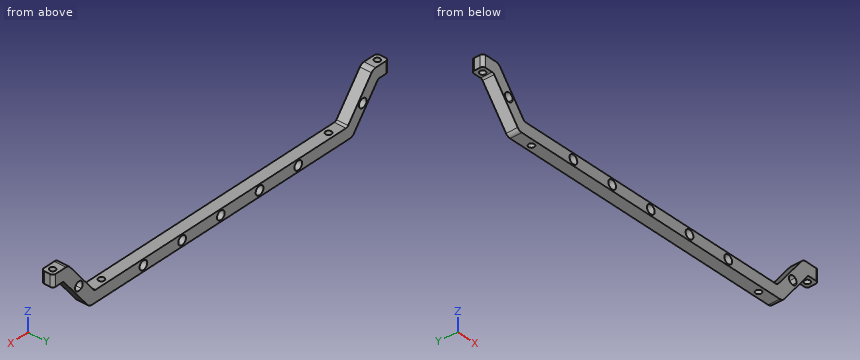
```python
from build123d import *

# Parameters (mm, degrees)
F0_R     = 7.5
F1_DEPTH = 10
F2_R     = 5
F5_D     = 10


with BuildPart() as f1:
    # F0 (on Front) → F1 (new body, symmetric)
    with BuildSketch(Plane.XZ):
        with BuildLine():
            Line((0, 10), (-245.075985, 10))
            Line((-245.075985, 10), (-242.07376, 6.097108))
            ThreePointArc((-242.07376, 6.097108), (-241.028627, -4.417518), (-250, -10))
            Line((-250, -10), (0, -10))
            Line((0, -10), (250, -10))
            ThreePointArc((250, -10), (241.028627, -4.417518), (242.07376, 6.097108))
            Line((242.07376, 6.097108), (245.075985, 10))
            Line((245.075985, 10), (0, 10))
        make_face()
        with Locations((-150, 0)):
            Circle(F0_R, mode=Mode.SUBTRACT)
        with BuildLine():
            ThreePointArc((-82.5, 0), (-75, 7.5), (-67.5, 0))
            ThreePointArc((-67.5, 0), (-75, -7.5), (-82.5, 0))
        make_face(mode=Mode.SUBTRACT)
        with BuildLine():
            ThreePointArc((7.5, 0), (0, -7.5), (-7.5, 0))
            ThreePointArc((-7.5, 0), (0, 7.5), (7.5, 0))
        make_face(mode=Mode.SUBTRACT)
        with BuildLine():
            ThreePointArc((82.5, 0), (75, -7.5), (67.5, 0))
            ThreePointArc((67.5, 0), (75, 7.5), (82.5, 0))
        make_face(mode=Mode.SUBTRACT)
        with BuildLine():
            ThreePointArc((157.5, 0), (150, -7.5), (142.5, 0))
            ThreePointArc((142.5, 0), (150, 7.5), (157.5, 0))
        make_face(mode=Mode.SUBTRACT)
        with BuildLine():
            ThreePointArc((-300, 75), (-308.971373, 69.417518), (-307.92624, 58.902892))
            Line((-307.92624, 58.902892), (-304.924015, 55))
            Line((-304.924015, 55), (-257.92624, -6.097108))
            ThreePointArc((-257.92624, -6.097108), (-254.417518, -8.971373), (-250, -10))
            ThreePointArc((-250, -10), (-241.028627, -4.417518), (-242.07376, 6.097108))
            Line((-242.07376, 6.097108), (-245.075985, 10))
            Line((-245.075985, 10), (-292.07376, 71.097108))
            ThreePointArc((-292.07376, 71.097108), (-295.582482, 73.971373), (-300, 75))
        make_face()
        with BuildLine():
            ThreePointArc((-270.427169, 26.55532), (-280.94468, 27.927169), (-279.572831, 38.44468))
            ThreePointArc((-279.572831, 38.44468), (-271.686862, 39.22853), (-267.5, 32.5))
            ThreePointArc((-267.5, 32.5), (-268.27147, 29.186862), (-270.427169, 26.55532))
        make_face(mode=Mode.SUBTRACT)
        with BuildLine():
            Line((-304.924015, 55), (-307.92624, 58.902892))
            ThreePointArc((-307.92624, 58.902892), (-308.971373, 69.417518), (-300, 75))
            Line((-300, 75), (-320, 75))
            Line((-320, 75), (-325.074017, 75))
            Line((-325.074017, 75), (-325.074017, 55))
            Line((-325.074017, 55), (-320, 55))
            Line((-320, 55), (-319.222152, 55))
            Line((-319.222152, 55), (-304.924015, 55))
        make_face()
        with BuildLine():
            Line((292.07376, 71.097108), (245.075985, 10))
            Line((245.075985, 10), (242.07376, 6.097108))
            ThreePointArc((242.07376, 6.097108), (241.028627, -4.417518), (250, -10))
            ThreePointArc((250, -10), (254.417518, -8.971373), (257.92624, -6.097108))
            Line((257.92624, -6.097108), (304.924015, 55))
            Line((304.924015, 55), (307.92624, 58.902892))
            ThreePointArc((307.92624, 58.902892), (308.971373, 69.417518), (300, 75))
            ThreePointArc((300, 75), (295.582482, 73.971373), (292.07376, 71.097108))
        make_face()
        with BuildLine():
            ThreePointArc((279.572831, 38.44468), (281.72853, 35.813138), (282.5, 32.5))
            ThreePointArc((282.5, 32.5), (278.313138, 25.77147), (270.427169, 26.55532))
            ThreePointArc((270.427169, 26.55532), (269.05532, 37.072831), (279.572831, 38.44468))
        make_face(mode=Mode.SUBTRACT)
        with BuildLine():
            Line((320, 75), (300, 75))
            ThreePointArc((300, 75), (308.971373, 69.417518), (307.92624, 58.902892))
            Line((307.92624, 58.902892), (304.924015, 55))
            Line((304.924015, 55), (319.222152, 55))
            Line((319.222152, 55), (320, 55))
            Line((320, 55), (325.074017, 55))
            Line((325.074017, 55), (325.074017, 75))
            Line((325.074017, 75), (320, 75))
        make_face()
    extrude(amount=F1_DEPTH, both=True)

    # F2
    f2_edges = [f1.edges().sort_by_distance(p)[0] for p in [
        (-245.075985, 0, 10),
        (245.075985, 0, 10),
        (-304.924015, 0, 55),
        (-325.074017, 10, 65),
        (325.074017, -10, 65),
        (325.074017, 10, 65),
        (-325.074017, -10, 65),
    ]]
    fillet(f2_edges, radius=F2_R)

    # F5 (through all)
    with Locations(Plane(origin=(0, 0, -10), x_dir=(1, 0, 0), z_dir=(0, 0, -1))):
        with Locations((-220, 0), (220, 0), (314.522654, 0), (-314.522654, 0)):
            Hole(F5_D / 2)


solid = f1.part
```
Design review of the part built by this model. Coordinates are the model's own, in mm. Coordinates: 2 decimals unless noted, no trailing zeros. Write each loop counter-clockwise with the first axis right and the second up, starting at its lowest first coordinate (ties: lowest second). Pieces come first, ordered by that corner, then holes.
1) Add section A-A (z = 0). Write out the cut boundary in (x, y), plus the area to 3 significant figures.
2) To check wall thickness, follow L1, parallel to Z at x = 75, y = 3.75; L2, parallel to Y at x = 220, z = -1; L3, parallel to X at y = -6.5, z = 2. State the ranges of each line that lie inside material, in increasing order.
3) Insertion check: pin 1 (4 mm diameter, centred on y = -4, z = 17.5, fed in from -X); pin 2 (10 mm diameter, centred on x = 319.5, y = 2, fed in from -Z); pin 3 (8 mm diameter, centred on x = -17.5, y = -7.5, fed in from +Z). Each pin has a flat end and moves straight along its axis. Give the tip position at first contact, or say it passes through.
4) Add section B-B (x = 150). Write out the cut boundary in (y, z), plus the area to 3 significant figures.
Check result:
1. outline: (-262.62, -10) - (-157.5, -10) - (-157.5, 10) - (-262.62, 10) - close; (-142.5, -10) - (-82.5, -10) - (-82.5, 10) - (-142.5, 10) - close; (-67.5, -10) - (-7.5, -10) - (-7.5, 10) - (-67.5, 10) - close; (7.5, -10) - (67.5, -10) - (67.5, 10) - (7.5, 10) - close; (82.5, -10) - (142.5, -10) - (142.5, 10) - (82.5, 10) - close; (157.5, -10) - (262.62, -10) - (262.62, 10) - (157.5, 10) - close; hole circle Ø10 at (-220, 0); hole circle Ø10 at (220, 0)
1. area: 8,850 mm2
2. L1: z = -10 to -7.5, 7.5 to 10
2. L2: y = -10 to -5, 5 to 10
2. L3: x = -264.15 to -157.23, -142.77 to -82.23, -67.77 to -7.23, 7.23 to 67.77, 82.23 to 142.77, 157.23 to 264.15
3. pin 1: stops at x = -277.62
3. pin 2: stops at z = 55
3. pin 3: stops at z = 10
4. outline: (-10, -10) - (10, -10) - (10, -7.5) - (-10, -7.5) - close; (-10, 7.5) - (10, 7.5) - (10, 10) - (-10, 10) - close
4. area: 100 mm2
